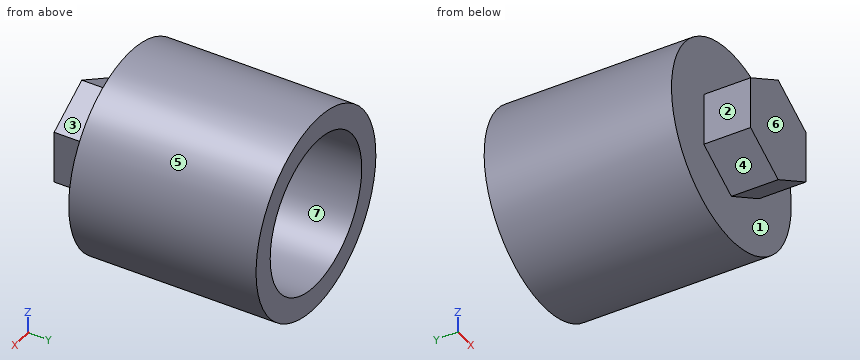
from build123d import *

# Parameters (mm, degrees)
SKETCH1_R                   = 13.5
BOSS_EXTRUDE1_DEPTH         = 25.4
F_7_8_14_TAPPED_HOLE1_D     = 20.6375
F_7_8_14_TAPPED_HOLE1_DEPTH = 19.05
F_7_8_14_TAPPED_HOLE1_TIP   = 6.200130513
BOSS_EXTRUDE2_DEPTH         = 6.35


with BuildPart() as part:
    # Sketch1 → Boss-Extrude1 (new body)
    with BuildSketch(Plane(origin=(0, 0, 0), x_dir=(1, 0, 0), z_dir=(0, 1, 0))):
        with Locations(Location((0, 0, 0), (0, 0, 270))):
            Circle(SKETCH1_R)
    extrude(amount=BOSS_EXTRUDE1_DEPTH)

    # 7/8-14 Tapped Hole1
    with Locations(Plane(origin=(0, 25.4, 0), x_dir=(1, 0, 0), z_dir=(0, 1, 0))):
        with Locations((0, 0)):
            Hole(F_7_8_14_TAPPED_HOLE1_D / 2, depth=F_7_8_14_TAPPED_HOLE1_DEPTH)
            with Locations((0, 0, -(F_7_8_14_TAPPED_HOLE1_DEPTH + F_7_8_14_TAPPED_HOLE1_TIP / 2))):  # 118° drill point
                Cone(0, F_7_8_14_TAPPED_HOLE1_D / 2, F_7_8_14_TAPPED_HOLE1_TIP, mode=Mode.SUBTRACT)

    # Sketch6 → Boss-Extrude2 (add)
    with BuildSketch(Plane.XZ):
        Polygon((6.223, 3.592850725), (0, 7.18570145), (-6.223, 3.592850725), (-6.223, -3.592850725), (0, -7.18570145), (6.223, -3.592850725), align=None)
    extrude(amount=BOSS_EXTRUDE2_DEPTH)


solid = part.part
Geometry check sheet. Reference: the model listing, model coordinates, mm. Face numbers are marked on the shaded views. A direction names the side the tool comes from. Give positions to 0.01 mm unless a question says otherwise; leave off trailing zeros. Order: outer loops, then holes, each group sorted by start corner. A loop starts at its lowest first (then second) coordinate and runs counter-clockwise, first axis right, second up.
1. Access from +Z, -Z, +X, -X, +Y, -Y to the whole of each face (thin tool, end or side, straight path). Record for the marked faces 1, 2 and 3.
Completed:
face 1: -Y
face 2: +Z, -Z, -X, -Y
face 3: +Z, +X, -Y
2. Depth check by flat-ended pin: pin 1 (1 mm diameter, centred on x = 3.5, y = 13, fed in from +Z); pin 2 (4 mm diameter, centred on x = -3.5, y = 0, fed in from +Z); pin 3 (6 mm diameter, centred on y = 10.5, z = 8, fed in from -X). Enter the tip coordinate at first touch or a pass-through.
Completed:
pin 1: stops at z = 13.16
pin 2: stops at z = 13.42
pin 3: stops at x = -12.54
3. Sectioned sample at B-B (x = 11.5). Record the boundary of the cut face in (y, z).
Completed:
outline: (0, -7.07) - (25.4, -7.07) - (25.4, 7.07) - (0, 7.07) - close
4. Draft check along Z on the marked faces 4, 5, 6 and 7. Enter one of: pulls with the +Z half, pulls with the -Z half, needs draft (parallel to the pull), parting line crosses it, or undercut.
Completed:
face 4: pulls with the -Z half
face 5: parting line crosses it
face 6: needs draft
face 7: undercut
5. Sectioned sample at A-A (y = 8). Record the boundary of the cut face in (x, z).
Completed:
outline: circle Ø27 at (0, 0); hole circle Ø20.64 at (0, 0)
6. Sectioned sample at C-C (z = 11). Record the boundary of the cut face in (x, y), then the cut area to 3 significant figures.
Completed:
outline: (-7.83, 0) - (7.83, 0) - (7.83, 25.4) - (-7.83, 25.4) - close
area: 398 mm2
7. Scan lines: line 1 (Z direction, x = -1.75, y = 5.5); line 2 (X direction, y = 12, z = 7.5); line 3 (X direction, y = 10, z = -1.75). Record each from-to range of solid material in increasing order.
Completed:
line 1: z = -13.39 to -8.73, 8.73 to 13.39
line 2: x = -11.22 to -7.09, 7.09 to 11.22
line 3: x = -13.39 to -10.17, 10.17 to 13.39
